from build123d import *

# Parameters (mm, degrees)
F1_DEPTH = 12.7
F2_R     = 3.254068
F3_DEPTH = 12.701


with BuildPart() as f1:
    # F0 (on Front) → F1 (new body)
    with BuildSketch(Plane.XZ):
        Polygon((-26.135963, 56.065113), (-48.990875, 55.815339), (-4.400152, -28.386429), (0, -28.386429), (35.437245, 36.122989), (60.109265, 36.122989), (70.294961, 56.041688), (-23.639806, 56.041688), (-13.454107, 36.802039), (13.481406, 36.802039), (-1.910316, 10.319223), align=None)
    extrude(amount=F1_DEPTH)

    # F2 (on face) → F3 (cut, through all)
    with BuildSketch(Plane.XZ.offset(12.7)):
        with Locations((61.512932, 51.409215)):
            Circle(F2_R)
    extrude(amount=-F3_DEPTH, mode=Mode.SUBTRACT)


solid = f1.part
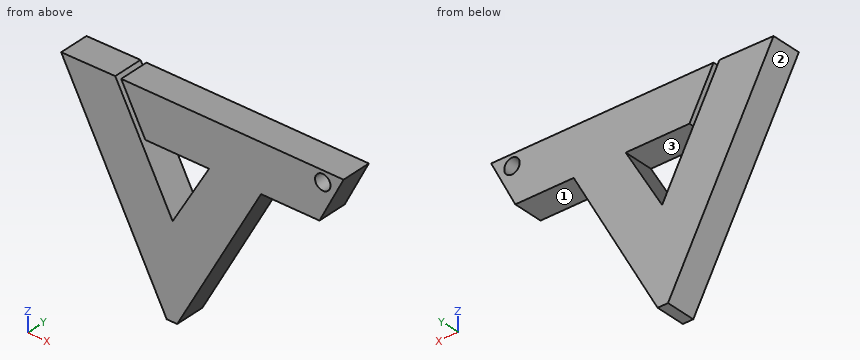
Can you work these out from the model? Positions are in its coordinate system, mm. Face numbers are marked on the shaded views. Coordinates: 2 decimals unless noted, no trailing zeros. Order: outer loops, then holes, each group sorted by start corner. A loop starts at its lowest first (then second) coordinate and runs counter-clockwise, first axis right, second up. Notation, with made-up numbers: M -32,66 L 4,66 A8 cw 4,76 Z; hole C 16.25,-4.5 d4. An arc over 180 degrees is marked long. Write item = value, one per line.
(1) Suppose I cut it at A-A on y = -3. Please give me the cut outline in (x, z).
Results are:
outline = M -48.99,55.82 L -4.4,-28.39 L 0,-28.39 L 35.44,36.12 L 60.11,36.12 L 70.29,56.04 L -23.64,56.04 L -13.45,36.8 L 13.48,36.8 L -1.91,10.32 L -26.14,56.07 Z; hole C 61.51,51.41 d6.51
(2) I need wall thicknesses on line 1 along Z through (x, y) = (35.5, -11); line 2 along X through (y, z) = (-3.5, 24.5); line 3 along X through (y, z) = (-6, 42). Which ranges of each line are inside material? Lowest first, please. Write a range as [from, to].
Results are:
line_1 = [36.12, 56.04]
line_2 = [-32.41, -9.42], [6.33, 29.05]
line_3 = [-41.67, -18.69], [-16.21, 63.11]
(3) For pin 1 Ø10.5 at (x, z) = (61.51, 51.41) entering from +Y; pin 2 Ø3 at (y, z) = (-8.5, 1) entering from -X; pin 3 Ø1 at (y, z) = (-5.5, -16) entering from +X; pin 4 Ø1.5 at (y, z) = (-4.5, 4.5) entering from +X, each with a flat end and sliding along its axis, tell me the tip position at first contact or that it passes through.
Results are:
pin_1 = 0
pin_2 = -20.76
pin_3 = 7.08
pin_4 = 18.48
(4) If we mould it in two halves opening along X, with no side actions, what happens to the marked faces 1, 2 and 3? For each: pulls with the +X half, pulls with the -X half, needs draft (parallel to the pull), parting line crosses it, or undercut.
Results are:
face_1 = needs draft
face_2 = pulls with the -X half
face_3 = undercut
(5) Suppose I cut it at D-D on z = 32. Please give me the cut outline in (x, y).
Results are:
outline = M -36.38,-12.7 L -13.39,-12.7 L -13.39,0 L -36.38,0 Z; M 10.69,-12.7 L 33.17,-12.7 L 33.17,0 L 10.69,0 Z
(6) Suppose I cut it at C-C on x = 5. Please give me the cut outline in (y, z), plus the area to 3 significant figures.
Results are:
outline = M -12.7,-19.28 L 0,-19.28 L 0,22.21 L -12.7,22.21 Z; M -12.7,36.8 L 0,36.8 L 0,56.04 L -12.7,56.04 Z
area = 771 mm2
(7) Suppose I cut it at B-B on z = 50. Please give me the cut outline in (x, y), plus the area to 3 significant figures.
Results are:
outline = M -45.91,-12.7 L -22.92,-12.7 L -22.92,0 L -45.91,0 Z; M -20.44,-12.7 L 58.58,-12.7 L 58.58,0 L -20.44,0 Z; M 64.45,-12.7 L 67.21,-12.7 L 67.21,0 L 64.45,0 Z
area = 1,330 mm2
